```python
from build123d import *

# Parameters (mm, degrees)
SKETCH1_R           = 12.5
BOSS_EXTRUDE1_DEPTH = 350
SKETCH3_R           = 15
SKETCH2_R           = 14
SKETCH4_W           = 8
SKETCH4_H           = 37
CUT_EXTRUDE2_DEPTH  = 7


with BuildPart() as part:
    # Sketch1 → Boss-Extrude1 (new body)
    with BuildSketch(Plane.YZ):
        with Locations(Location((0, 0, 0), (0, 0, 270))):
            Circle(SKETCH1_R)
    extrude(amount=BOSS_EXTRUDE1_DEPTH)

    # Sketch3 → Loft1 section 0
    with BuildSketch(Plane.YZ.offset(100)):
        Circle(SKETCH3_R)
    # Sketch2 → Loft1 section 1
    with BuildSketch(Plane.YZ.offset(80)):
        Circle(SKETCH2_R)
    loft()

    # Sketch4 → Cut-Extrude2 (cut)
    with BuildSketch(Plane(origin=(0, 0, 10), x_dir=(0, 1, 0), z_dir=(0, 0, 1))):
        with Locations((0.007753839, -118.5)):
            Rectangle(SKETCH4_W, SKETCH4_H)
    extrude(amount=-CUT_EXTRUDE2_DEPTH, mode=Mode.SUBTRACT)


solid = part.part
```
Build history of the part. All positions in model axes, mm. A direction names the side the tool comes from. Coordinates: 2 decimals unless noted, no trailing zeros. Order: outer loops, then holes, each group sorted by start corner. A loop starts at its lowest first (then second) coordinate and runs counter-clockwise, first axis right, second up. Notation, with made-up numbers: M 51.5,-31.75 L 62.5,-31.75 A23 cw 62.5,3.25 Z; hole C 68,14.5 d3. An arc over 180 degrees is marked long. One line per question, with ' | ' between items. Start each with the question number.
1. Cut at B-B (x = 319). Write the cut outline in (y, z).
2. Cut at A-A (y = 0). Write the cut outline in (x, z), plus the area to 3 significant figures.
3. Wall check: line 1 along Z through (x, y) = (115, 1); line 2 along X through (y, z) = (-3.5, 8.5); line 3 along Y through (x, z) = (241, 0). Give the ranges that are in metal, low to high. Write a range as [from, to].
4. Mould opens along X. For faces 1 (the face through (350, 0, 0)), 2 (the face through (89.86, -3.14, -14.15)), 3 (the face through (118, 0, 10)), 4 (the face through (100, 0, 7)) say: +X half, -X half, draft (parallel to the pull), parting line (faces both ways), or undercut.
5. Tool access for faces 5 (the face through (0, 0, 0)), 6 (the face through (39.44, 3.755, -11.923)), 7 (the face through (100, -3.4, 12.3)), 8 (the face through (119, 4.008, 7)): list every direction of +Z, -Z, +X, -X, +Y, -Y with a clear straight run to the whole face (end or side of a thin tool).
6. Flat gauge pins, fed straight in: P1, Ø3, axis at x = 193, y = -5.5, coming from the +Z side; P2, Ø2, axis at x = 114, z = 5.5, coming from the +Y side; P3, Ø2.5, axis at x = 118.5, y = -2, coming from the +Z side. Where does each tip first touch, or does it go through?
The answers:
1) outline: C 0,0 d25
2) outline: M 0,-12.5 L 80,-12.5 L 80,-14 L 100,-15 L 100,-12.5 L 350,-12.5 L 350,12.5 L 100,12.5 L 100,15 L 80,14 L 80,12.5 L 0,12.5 Z; hole M 100,3 L 137,3 L 137,10 L 100,10 Z | area: 8,570 mm2
3) line 1: z = [-12.46, 3], [10, 12.46] | line 2: x = [0, 100], [137, 350] | line 3: y = [-12.5, 12.5]
4) face 1: +X half | face 2: -X half | face 3: undercut | face 4: undercut
5) face 5: +Z, -Z, -X, +Y, -Y | face 6: -X | face 7: +X | face 8: none
6) P1: stops at z = 11.84 | P2: stops at y = 11.66 | P3: stops at z = 12.48
